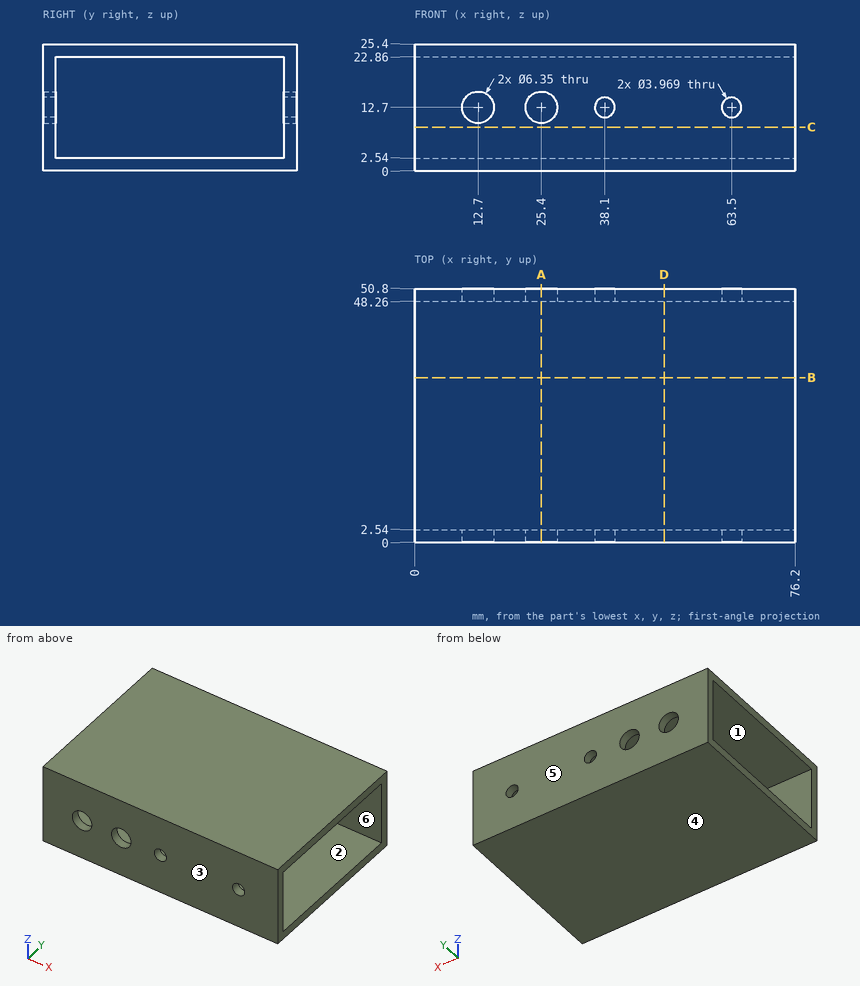
Drawing for the job (mm, zero at the part's lowest x, y, z). A direction names the side the tool comes from. Round coordinates to 2 decimals unless told otherwise and drop trailing zeros. Order: outer loops, then holes, each group sorted by start corner. A loop starts at its lowest first (then second) coordinate and runs counter-clockwise, first axis right, second up. Notation, with made-up numbers: (-32.75, 30) -> (21.25, 30) arc R34 ccw to (21.25, 61) -> close; hole circle Ø5 at (65, 72.25). An arc over 180 degrees is marked (long way). Write item = value, one per line. Start each with the question number.
(1) Probe line 1 (X direction, y = 50.1, z = 12.7) (1 decimal); line 2 (Y direction, x = 5, z = 20.75); line 3 (Z direction, x = 63.5, y = 1.65). List the from-to ranges inside material, lowest first. Write a range as [from, to].
(2) Pull direction Y, two halves, no side cores. Call the marked faces 1, 2, 3 and 4: released by +Y, released by -Y, zero draft, split by the parting line, or undercut.
(3) Cut at A-A, the plane x = 25.4. List the corners of the cut face in (y, z) (3 decimals), then the cut area to 3 significant figures.
(4) Which spindle directions (+Z, -Z, +X, -X, +Y, -Y) get a long thin tool onto all of the face, cutting with end or side? Do the marked faces 5 and 6. Say none if no direction does.
(5) Cut at B-B, the plane y = 33. List the corners of the cut face in (x, z).
(6) Cut at D-D, the plane x = 50. List the corners of the cut face in (y, z).
(7) Cut at C-C, the plane z = 8.75. List the corners of the cut face in (x, y), then the cut area to 3 significant figures.
Model answer:
q1.line_1 = [0, 9.5], [15.9, 22.2], [28.6, 36.1], [40.1, 61.5], [65.5, 76.2]
q1.line_2 = [0, 2.54], [48.26, 50.8]
q1.line_3 = [0, 10.72], [14.68, 25.4]
q2.face_1 = undercut
q2.face_2 = undercut
q2.face_3 = released by -Y
q2.face_4 = zero draft
q3.outline = (0, 0) -> (50.8, 0) -> (50.8, 9.525) -> (48.26, 9.525) -> (48.26, 2.54) -> (2.54, 2.54) -> (2.54, 9.525) -> (0, 9.525) -> close; (0, 15.875) -> (2.54, 15.875) -> (2.54, 22.86) -> (48.26, 22.86) -> (48.26, 15.875) -> (50.8, 15.875) -> (50.8, 25.4) -> (0, 25.4) -> close
q3.area = 329 mm2
q4.face_5 = +Z, -Z, +X, -X, +Y
q4.face_6 = +X, -X
q5.outline = (0, 0) -> (76.2, 0) -> (76.2, 2.54) -> (0, 2.54) -> close; (0, 22.86) -> (76.2, 22.86) -> (76.2, 25.4) -> (0, 25.4) -> close
q6.outline = (0, 0) -> (50.8, 0) -> (50.8, 25.4) -> (0, 25.4) -> close; hole (2.54, 2.54) -> (48.26, 2.54) -> (48.26, 22.86) -> (2.54, 22.86) -> close
q7.outline = (0, 0) -> (76.2, 0) -> (76.2, 2.54) -> (0, 2.54) -> close; (0, 48.26) -> (76.2, 48.26) -> (76.2, 50.8) -> (0, 50.8) -> close
q7.area = 387 mm2
